The listing builds one solid part. Answer for the finished solid, in the listing's coordinates (mm). Face numbers are marked on the shaded views. A direction names the side the tool comes from. Coordinates: 2 decimals unless noted, no trailing zeros. Write each loop counter-clockwise with the first axis right and the second up, starting at its lowest first coordinate (ties: lowest second). Pieces come first, ordered by that corner, then holes.
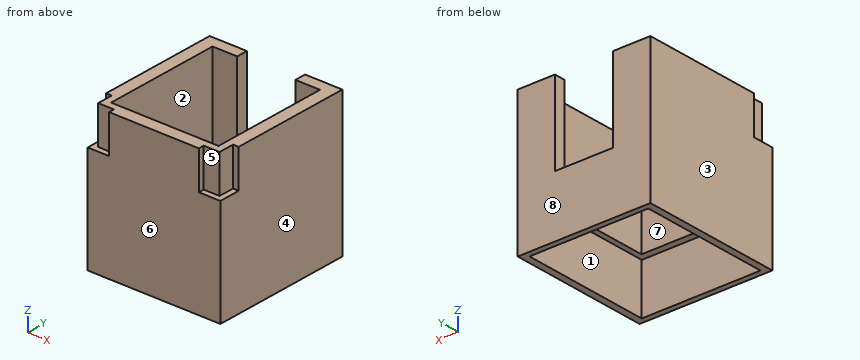
from build123d import *

# Parameters (mm, degrees)
SKETCH112_W     = 52.5
SKETCH112_H     = 56.5
SKETCH112_W_2   = 42.5
SKETCH112_H_2   = 47
PAD058_DEPTH    = 37
SKETCH113_W     = 23
SKETCH113_H     = 33
POCKET050_DEPTH = 5
SKETCH114_W     = 52.5
SKETCH114_H     = 56.5
SKETCH114_W_2   = 47
SKETCH114_H_2   = 52
PAD059_DEPTH    = 20
POCKET060_DEPTH = 15


with BuildPart() as part:
    # Sketch112 → Pad058 (new body)
    with BuildSketch(Plane.XY):
        with Locations((0, -26)):
            Rectangle(SKETCH112_W, SKETCH112_H)
        with Locations((0, -25.75)):
            Rectangle(SKETCH112_W_2, SKETCH112_H_2, mode=Mode.SUBTRACT)
    extrude(amount=PAD058_DEPTH)

    # Sketch113 (on Face1 of Pad058) → Pocket050 (cut)
    with BuildSketch(Plane(origin=(0, 2.25, 0), x_dir=(-1, 0, 0), z_dir=(0, 1, 0))):
        with Locations((0, 20.5)):
            Rectangle(SKETCH113_W, SKETCH113_H)
    extrude(amount=-POCKET050_DEPTH, mode=Mode.SUBTRACT)

    # Sketch114 (on Face2 of Pocket050) → Pad059 (join)
    with BuildSketch(Plane(origin=(0, 0, 0), x_dir=(1, 0, 0), z_dir=(0, 0, -1))):
        with Locations((0, 26)):
            Rectangle(SKETCH114_W, SKETCH114_H)
        with Locations((0, 26)):
            Rectangle(SKETCH114_W_2, SKETCH114_H_2, mode=Mode.SUBTRACT)
    extrude(amount=PAD059_DEPTH)

    # Sketch136 (on Face1 of Pad059) → Pocket060 (cut)
    with BuildSketch(Plane.XY.offset(37)):
        Polygon((-26.25, -54.25), (-26.25, -45.75), (-24, -45.75), (-24, -52), (-17.75, -52), (-17.75, -54.25), align=None)
        Polygon((26.25, -54.25), (26.25, -45.75), (24, -45.75), (24, -52), (17.75, -52), (17.75, -54.25), align=None)
    extrude(amount=-POCKET060_DEPTH, mode=Mode.SUBTRACT)


with BuildPart() as part_1:
    # Body032 placement: moved
    add(part.part.moved(Location((0, 0, 135))))


solid = part_1.part
Q1. Which of the six approach directions +Z, -Z, +X, -X, +Y, -Y give full straight-line access (tool end or side, diameter ignored) to the marked faces 1, 2, 3, 4 and 5?
Answers below:
face 1: -Z
face 2: +Z, -Z
face 3: +Z, -Z, -X, +Y, -Y
face 4: +Z, -Z, +X, +Y, -Y
face 5: +Z, +X, -Y
Q2. The part is cut by section C-C, the plane y = -38. Write down the section's boundary in (x, z), then the cut area to 3 significant figures.
Answers below:
outline: (-26.25, 115) - (-23.5, 115) - (-23.5, 135) - (-21.25, 135) - (-21.25, 172) - (-26.25, 172) - close; (21.25, 135) - (23.5, 135) - (23.5, 115) - (26.25, 115) - (26.25, 172) - (21.25, 172) - close
area: 480 mm2
Q3. The part is cut by section B-B, the plane z = 131.5. Write down the section's boundary in (x, y).
Answers below:
outline: (-26.25, -54.25) - (26.25, -54.25) - (26.25, 2.25) - (-26.25, 2.25) - close; hole (-23.5, -52) - (23.5, -52) - (23.5, 0) - (-23.5, 0) - close
Q4. The part is cut by section A-A, the plane x = 13. Write down the section's boundary in (y, z), then the cut area to 4 significant figures.
Answers below:
outline: (-54.25, 115) - (-52, 115) - (-52, 135) - (-49.25, 135) - (-49.25, 172) - (-54.25, 172) - close; (-2.25, 135) - (0, 135) - (0, 115) - (2.25, 115) - (2.25, 172) - (-2.25, 172) - close
area: 441.5 mm2
Q5. Determine the mould class of the marked faces 6, 7 and 8 for opening direction Y: released by +Y, released by -Y, zero draft, split by the parting line, or undercut.
Answers below:
face 6: released by -Y
face 7: undercut
face 8: released by +Y
Q6. The part is cut by section D-D, the plane z = 146.5. Write down the section's boundary in (x, y).
Answers below:
outline: (-26.25, -54.25) - (26.25, -54.25) - (26.25, 2.25) - (11.5, 2.25) - (11.5, -2.25) - (21.25, -2.25) - (21.25, -49.25) - (-21.25, -49.25) - (-21.25, -2.25) - (-11.5, -2.25) - (-11.5, 2.25) - (-26.25, 2.25) - close
Q7. Given pin 1 (1.9 mm diameter, centred on y = -50, z = 166.5, fed in from +X); pin 2 (2 mm diameter, centred on x = 20, y = -9.5, fed in from +Z); pin 3 (12 mm diameter, centred on x = -4, y = -47, fed in from -Z); pin 4 (5 mm diameter, centred on x = -22, z = 162, fed in from -Y), each flat-ended and moving along its own axis, determine where each tip first touches the part or whether it passes through.
Answers below:
pin 1: stops at x = 24
pin 2: passes through
pin 3: stops at z = 115
pin 4: stops at y = -52
Q8. Find the intervals of material crossed by probe 1 along X at (y, z) = (-26.5, 147); probe 2 along Y at (x, z) = (13.5, 152); probe 3 along Y at (x, z) = (10.5, 127), in increasing order.
Answers below:
probe 1: x = -26.25 to -21.25, 21.25 to 26.25
probe 2: y = -54.25 to -49.25, -2.25 to 2.25
probe 3: y = -54.25 to -52, 0 to 2.25
